Design review of the part shown in the three views and the two pictorial views. Dimensions are in mm from the part's minimum x, y and z. Give positions to 0.01 mm unless a question says otherwise; leave off trailing zeros. Loops run counter-clockwise (first coordinate to the right, second up) from the corner with the lowest first, then second, coordinate; pieces in that order, holes last.
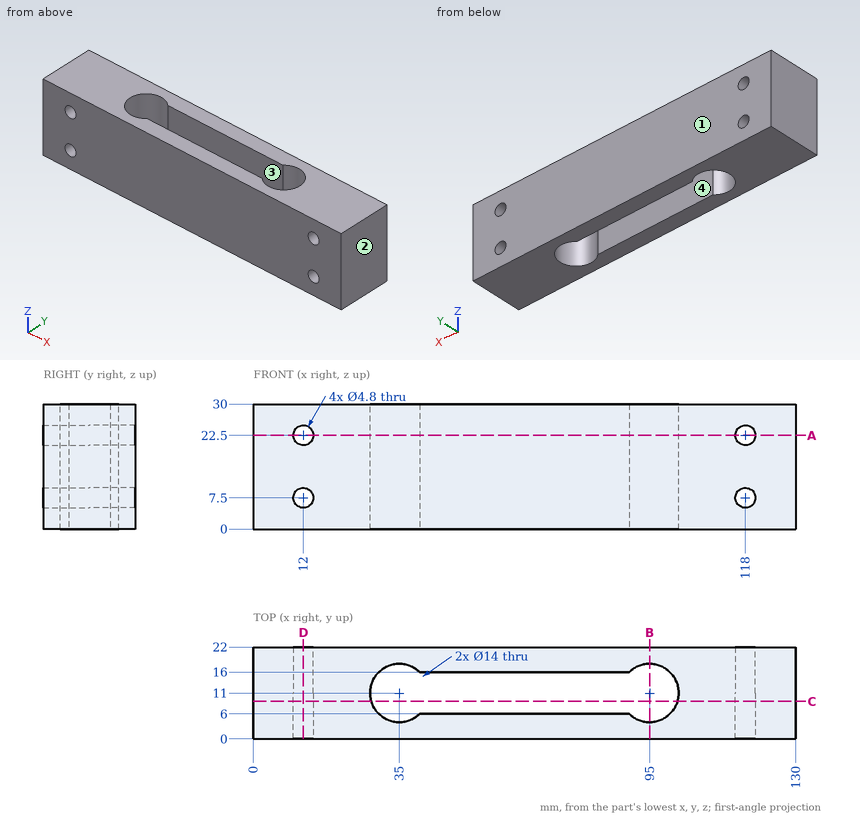
Q1. Consider section A-A on z = 22.5. Give the boundary of the cut face in (x, y), plus the area to 3 significant figures.
Answers:
outline: (0, 0) - (9.6, 0) - (9.6, 22) - (0, 22) - close; (14.4, 0) - (115.6, 0) - (115.6, 22) - (14.4, 22) - close; (120.4, 0) - (130, 0) - (130, 22) - (120.4, 22) - close; hole (39.9, 6) - (90.1, 6) arc R7 ccw (long way) to (90.1, 16) - (39.9, 16) arc R7 ccw (long way) to start
area: 1,870 mm2
Q2. Mouldability with a two-part tool opening along Y and no side actions: class the marked faces 1, 2, 3 and 4 as +Y half, -Y half, draft (parallel to the pull), parting line (faces both ways), or undercut.
Answers:
face 1: +Y half
face 2: draft
face 3: undercut
face 4: undercut
Q3. Consider section B-B on x = 95. Give the boundary of the cut face in (y, z), plus the area to 3 significant figures.
Answers:
outline: (0, 0) - (4, 0) - (4, 30) - (0, 30) - close; (18, 0) - (22, 0) - (22, 30) - (18, 30) - close
area: 240 mm2
Q4. For probe 1 along Z at (x, y) = (12, 14.5); probe 2 along X at (y, z) = (10.75, 18.25); probe 3 along Y at (x, z) = (35, 18.25), list the stretches that pass through material, from the lowest coordinate up.
Answers:
probe 1: z = 0 to 5.1, 9.9 to 20.1, 24.9 to 30
probe 2: x = 0 to 28, 102 to 130
probe 3: y = 0 to 4, 18 to 22
Q5. Consider section D-D on x = 12. Give the boundary of the cut face in (y, z), plus the area to 3 significant figures.
Answers:
outline: (0, 0) - (22, 0) - (22, 5.1) - (0, 5.1) - close; (0, 9.9) - (22, 9.9) - (22, 20.1) - (0, 20.1) - close; (0, 24.9) - (22, 24.9) - (22, 30) - (0, 30) - close
area: 449 mm2
Q6. Consider section C-C on y = 9. Give the boundary of the cut face in (x, z).
Answers:
outline: (0, 0) - (28.29, 0) - (28.29, 30) - (0, 30) - close; (101.71, 0) - (130, 0) - (130, 30) - (101.71, 30) - close; hole circle Ø4.8 at (12, 7.5); hole circle Ø4.8 at (12, 22.5); hole circle Ø4.8 at (118, 7.5); hole circle Ø4.8 at (118, 22.5)
